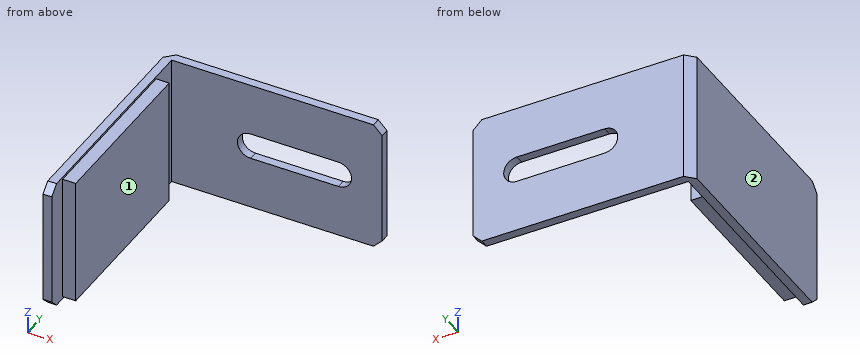
```python
from build123d import *

# Parameters (mm, degrees)
ESBO_O1_W                = 2
ESBO_O1_H                = 50
ESBO_O1_W_2              = 50
ESBO_O1_H_2              = 2
RESSALTO_EXTRUS_O1_DEPTH = 30
CHANFRO1_SIZE            = 2
ESBO_O2_R                = 3
ESBO_O2_W                = 20
ESBO_O2_H                = 6
CORTE_EXTRUS_O1_DEPTH    = 15
ESBO_O3_W                = 29
ESBO_O3_H                = 39
RESSALTO_EXTRUS_O2_DEPTH = 3


with BuildPart() as part:
    # Esboço1 → Ressalto-extrusão1 (new body)
    with BuildSketch(Plane.XY):
        with Locations((1, 25)):
            Rectangle(ESBO_O1_W, ESBO_O1_H)
        with Locations((25, 51)):
            Rectangle(ESBO_O1_W_2, ESBO_O1_H_2)
    extrude(amount=RESSALTO_EXTRUS_O1_DEPTH)

    # Chanfro1
    chanfro1_edges = [part.edges().sort_by_distance(p)[0] for p in [
        (1, 0, 0),
        (50, 51, 0),
        (0, 52, 15),
        (50, 51, 30),
        (1, 0, 30),
    ]]
    chamfer(chanfro1_edges, length=CHANFRO1_SIZE)

    # Esboço2 → Corte-extrusão1 (cut)
    with BuildSketch(Plane(origin=(0, 52, 0), x_dir=(1, 0, 0), z_dir=(0, 1, 0))):
        with Locations((40, -15)):
            Circle(ESBO_O2_R)
        with Locations((20, -15)):
            Circle(ESBO_O2_R)
        with Locations((30, -15)):
            Rectangle(ESBO_O2_W, ESBO_O2_H)
    extrude(amount=-CORTE_EXTRUS_O1_DEPTH, mode=Mode.SUBTRACT)

    # Esboço3 → Ressalto-extrusão2 (add)
    with BuildSketch(Plane(origin=(2, 0, 0), x_dir=(0, 0, -1), z_dir=(1, 0, 0))):
        with Locations((-15, 24)):
            Rectangle(ESBO_O3_W, ESBO_O3_H)
    extrude(amount=RESSALTO_EXTRUS_O2_DEPTH)


solid = part.part
```
Here's how the part is built. I have some questions about the finished solid (model axes, mm). Face numbers are marked on the shaded views. A direction names the side the tool comes from. Coordinates: 2 decimals unless noted, no trailing zeros. Write each loop counter-clockwise with the first axis right and the second up, starting at its lowest first coordinate (ties: lowest second). Pieces come first, ordered by that corner, then holes. Notation, with made-up numbers: (72, -14) - (106, -14) arc R7 ccw to (106, -7) - close; hole circle Ø11 at (61, -7.5). An arc over 180 degrees is marked (long way). One line per item, written item: value.
1) Suppose I cut it at A-A on z = 15. Write out the boundary of the cut face in (x, y).
Model answer:
outline: (0, 0) - (2, 0) - (2, 4.5) - (5, 4.5) - (5, 43.5) - (2, 43.5) - (2, 50) - (17, 50) - (17, 52) - (2, 52) - (0, 50) - close; (43, 50) - (50, 50) - (50, 52) - (43, 52) - close
2) I'm going to push flat-ended pins straight in: P1, Ø2.5, axis at x = 3.5, z = 15, coming from the -Y side; P2, Ø5, axis at y = 32.5, z = 12, coming from the +X side; P3, Ø1.5, axis at x = 4, y = 28.5, coming from the +Z side. Where does each tip first touch, or does it pass through?
Model answer:
P1: stops at y = 4.5
P2: stops at x = 5
P3: stops at z = 29.5
3) I need wall thicknesses on line 1 along Y through (x, z) = (15, 8); line 2 along Z through (x, y) = (4.5, 37); line 3 along X through (y, z) = (31, 15). Which ranges of each line are inside material? Lowest first, please.
Model answer:
line 1: y = 50 to 52
line 2: z = 0.5 to 29.5
line 3: x = 0 to 5
4) On a 3-axis mill with a long thin cutter (end or side, diameter ignored), from which of +Z, -Z, +X, -X, +Y, -Y can I reach the whole of each face in a straight line? I mean the marked faces 1 and 2. Say none if no direction works.
Model answer:
face 1: +Z, -Z, +X, -Y
face 2: +Z, -Z, -X, +Y, -Y
5) Suppose I cut it at B-B on z = 25. Write out the boundary of the cut face in (x, y), and give its area (3 significant figures).
Model answer:
outline: (0, 0) - (2, 0) - (2, 4.5) - (5, 4.5) - (5, 43.5) - (2, 43.5) - (2, 50) - (50, 50) - (50, 52) - (2, 52) - (0, 50) - close
area: 315 mm²
6) Suppose I cut it at D-D on x = 13. Write out the boundary of the cut face in (y, z).
Model answer:
outline: (50, 0) - (52, 0) - (52, 30) - (50, 30) - close
7) Suppose I cut it at C-C on y = 21. Write out the boundary of the cut face in (x, z).
Model answer:
outline: (0, 0) - (2, 0) - (2, 0.5) - (5, 0.5) - (5, 29.5) - (2, 29.5) - (2, 30) - (0, 30) - close
